Verification items for the finished model (mm, model axes). Face numbers are marked on the shaded views. A direction names the side the tool comes from. Coordinates: 2 decimals unless noted, no trailing zeros. Order: outer loops, then holes, each group sorted by start corner. A loop starts at its lowest first (then second) coordinate and runs counter-clockwise, first axis right, second up. Notation, with made-up numbers: M 89.25,51.25 L 116.25,51.25 A27 ccw 116.25,67.25 Z; hole C -22.5,62 d11. An arc over 180 degrees is marked long. Write item = value, one per line.
```python
from build123d import *

# Parameters (mm, degrees)
F1_DEPTH = 11.049
F2_DEPTH = 27.94
F3_DEPTH = 3.175
F4_R     = 9.525
F5_DEPTH = 2.54


with BuildPart() as f1:
    # F0 (on Front) → F1 (new body)
    with BuildSketch(Plane.XZ):
        with BuildLine():
            ThreePointArc((-32.0532864205, 3.175), (-32.9162675396, 5.2584207218), (-34.9996882613, 6.1214018409))
            Line((-34.9996882613, 6.1214018409), (-34.9996882613, 0.2285981591))
            ThreePointArc((-34.9996882613, 0.2285981591), (-32.9162675396, 1.0915792782), (-32.0532864205, 3.175))
        make_face()
        with BuildLine():
            Line((-34.9996882613, 0.2285981591), (-34.9996882613, 6.1214018409))
            ThreePointArc((-34.9996882613, 6.1214018409), (-37.9460901022, 3.175), (-34.9996882613, 0.2285981591))
        make_face()
    extrude(amount=F1_DEPTH)



with BuildPart() as f2:
    # F0 (on Front) → F2 (new body)
    with BuildSketch(Plane.XZ):
        with BuildLine():
            Line((46.2803117387, 0), (46.2803117387, 6.35))
            ThreePointArc((46.2803117387, 6.35), (43.1053117387, 3.175), (46.2803117387, 0))
        make_face()
        with BuildLine():
            ThreePointArc((49.4553117387, 3.175), (48.5253757689, 5.4200640303), (46.2803117387, 6.35))
            Line((46.2803117387, 6.35), (46.2803117387, 0))
            ThreePointArc((46.2803117387, 0), (48.5253757689, 0.9299359697), (49.4553117387, 3.175))
        make_face()
    extrude(amount=F2_DEPTH)


with BuildPart() as f1_1:
    add(f1.part)

    add(f2.part)  # F3 merges F2
    # F0 (on Front) → F3 (join, symmetric)
    with BuildSketch(Plane.XZ):
        with BuildLine():
            Line((46.2803117387, 6.35), (-34.9996882613, 6.35))
            ThreePointArc((-34.9996882613, 6.35), (-32.7546242311, 5.4200640303), (-31.8246882613, 3.175))
            ThreePointArc((-31.8246882613, 3.175), (-32.7546242311, 0.9299359697), (-34.9996882613, 0))
            Line((-34.9996882613, 0), (46.2803117387, 0))
            ThreePointArc((46.2803117387, 0), (43.1053117387, 3.175), (46.2803117387, 6.35))
        make_face()
        with BuildLine():
            Line((-34.9996882613, 6.1214018409), (-34.9996882613, 6.35))
            ThreePointArc((-34.9996882613, 6.35), (-38.1746882613, 3.175), (-34.9996882613, 0))
            Line((-34.9996882613, 0), (-34.9996882613, 0.2285981591))
            ThreePointArc((-34.9996882613, 0.2285981591), (-37.9460901022, 3.175), (-34.9996882613, 6.1214018409))
        make_face()
        with BuildLine():
            ThreePointArc((-31.8246882613, 3.175), (-32.7546242311, 5.4200640303), (-34.9996882613, 6.35))
            Line((-34.9996882613, 6.35), (-34.9996882613, 6.1214018409))
            ThreePointArc((-34.9996882613, 6.1214018409), (-32.9162675396, 5.2584207218), (-32.0532864205, 3.175))
            ThreePointArc((-32.0532864205, 3.175), (-32.9162675396, 1.0915792782), (-34.9996882613, 0.2285981591))
            Line((-34.9996882613, 0.2285981591), (-34.9996882613, 0))
            ThreePointArc((-34.9996882613, 0), (-32.7546242311, 0.9299359697), (-31.8246882613, 3.175))
        make_face()
        with BuildLine():
            ThreePointArc((49.4553117387, 3.175), (48.5253757689, 5.4200640303), (46.2803117387, 6.35))
            Line((46.2803117387, 6.35), (46.2803117387, 0))
            ThreePointArc((46.2803117387, 0), (48.5253757689, 0.9299359697), (49.4553117387, 3.175))
        make_face()
        with BuildLine():
            Line((46.2803117387, 0), (46.2803117387, 6.35))
            ThreePointArc((46.2803117387, 6.35), (43.1053117387, 3.175), (46.2803117387, 0))
        make_face()
        with BuildLine():
            Line((-34.9996882613, 0.2285981591), (-34.9996882613, 6.1214018409))
            ThreePointArc((-34.9996882613, 6.1214018409), (-37.9460901022, 3.175), (-34.9996882613, 0.2285981591))
        make_face()
        with BuildLine():
            ThreePointArc((-32.0532864205, 3.175), (-32.9162675396, 5.2584207218), (-34.9996882613, 6.1214018409))
            Line((-34.9996882613, 6.1214018409), (-34.9996882613, 0.2285981591))
            ThreePointArc((-34.9996882613, 0.2285981591), (-32.9162675396, 1.0915792782), (-32.0532864205, 3.175))
        make_face()
    extrude(amount=F3_DEPTH, both=True)

    # F4 (on face) → F5 (join)
    with BuildSketch(Plane.XZ.offset(27.94)):
        with Locations((46.2803117387, 3.175)):
            Circle(F4_R)
        with BuildLine():
            ThreePointArc((46.2803117387, 6.35), (48.5253757689, 5.4200640303), (49.4553117387, 3.175))
            ThreePointArc((49.4553117387, 3.175), (44.0352477084, 0.9299359697), (46.2803117387, 6.35))
        make_face(mode=Mode.SUBTRACT)
        with BuildLine():
            ThreePointArc((46.2803117387, 6.35), (44.0352477084, 0.9299359697), (49.4553117387, 3.175))
            ThreePointArc((49.4553117387, 3.175), (48.5253757689, 5.4200640303), (46.2803117387, 6.35))
        make_face()
    extrude(amount=F5_DEPTH)


solid = f1_1.part
```
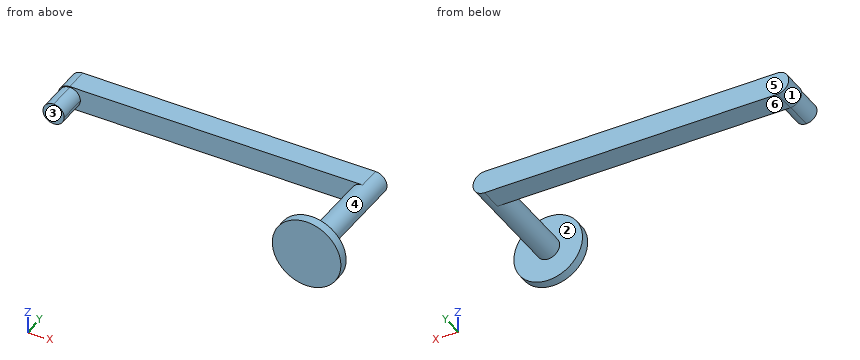
Item 1: Scan lines: L1, parallel to Z at x = -30, y = -1; L2, parallel to X at y = -11, z = 5; L3, parallel to X at y = -2, z = 3.5. Record each from-to range of solid material in increasing order. Write a range as from..to.
Report:
L1 = 0..6.35
L2 = -37.31..-32.69, 43.68..48.88
L3 = -38.16..49.44
Item 2: Tool access check on the marked faces 1, 2 and 3. Record the directions out of +Z, -Z, +X, -X, +Y, -Y that give a thin tool (end or side, any length) a straight path to the whole face; none if there is none.
Report:
face_1 = -X, +Y, -Y
face_2 = none
face_3 = +Z, -Z, -X, -Y
Item 3: Sectioned sample at B-B, the plane z = 4. Enter the section's corners in (x, y) (3 decimals).
Report:
outline = M -38.066,-3.175 L -37.828,-3.175 L -37.828,-11.049 L -32.171,-11.049 L -32.171,-3.175 L 43.214,-3.175 L 43.214,-27.94 L 36.791,-27.94 L 36.791,-30.48 L 55.77,-30.48 L 55.77,-27.94 L 49.346,-27.94 L 49.346,3.175 L -38.066,3.175 Z
Item 4: Sectioned sample at A-A, the plane x = 33. Enter the section's corners in (y, z) (3 decimals).
Report:
outline = M -3.175,0 L 3.175,0 L 3.175,6.35 L -3.175,6.35 Z
Item 5: Sectioned sample at C-C, the plane y = 1. Enter the section's corners in (x, z) (3 decimals), then the cut area to 3 significant figures.
Report:
outline = M -35,0 L 46.28,0 A3.175 ccw 46.28,6.35 L -35,6.35 A3.175 ccw Z
area = 548 mm^2
Item 6: Gauge pin test, flat ends, axial feed: pin 1 (3 mm diameter, centred on x = 22.5, z = 4, fed in from -Y) (3 decimals); pin 2 (1.5 mm diameter, centred on x = 4, z = 7, fed in from +Y) (3 decimals); pin 3 (5 mm diameter, centred on x = 13, y = -1.5, fed in from +Z); pin 4 (1.5 mm diameter, centred on x = 46.5, y = -2.5, fed in from -Z). Record the tip position at first contact, or that the pin passes through.
Report:
pin_1 = -3.175
pin_2 = 3.175
pin_3 = 6.35
pin_4 = 0
Item 7: Release check for a two-part mould opening along Y. For the marked faces 4, 5 and 6 record: pulls with the +Y half, pulls with the -Y half, needs draft (parallel to the pull), parting line crosses it, or undercut.
Report:
face_4 = undercut
face_5 = pulls with the +Y half
face_6 = needs draft
Item 8: Sectioned sample at D-D, the plane y = -20.5. Enter the section's corners in (x, z) (3 decimals).
Report:
outline = C 46.28,3.175 d6.35
